from build123d import *

# Parameters (mm, degrees)
SKETCH_W  = 50.56
SKETCH_H  = 128.5
SKETCH_R  = 1.6
PAD_DEPTH = 2


with BuildPart() as part:
    # Sketch → Pad (new body)
    with BuildSketch(Plane.XZ):
        Rectangle(SKETCH_W, SKETCH_H)
        with Locations((-17.78, 61.25)):
            Circle(SKETCH_R, mode=Mode.SUBTRACT)
        with Locations((17.78, 61.25)):
            Circle(SKETCH_R, mode=Mode.SUBTRACT)
        with Locations((17.78, -61.25)):
            Circle(SKETCH_R, mode=Mode.SUBTRACT)
        with Locations((-17.78, -61.25)):
            Circle(SKETCH_R, mode=Mode.SUBTRACT)
    extrude(amount=PAD_DEPTH)


solid = part.part
Here's how the part is built. I have some questions about the finished solid (model axes, mm). Round coordinates to 2 decimals unless told otherwise and drop trailing zeros. Order: outer loops, then holes, each group sorted by start corner. A loop starts at its lowest first (then second) coordinate and runs counter-clockwise, first axis right, second up. Notation, with made-up numbers: (6.25, 6) -> (28.25, 6) arc R17 ccw to (28.25, 14) -> close; hole circle Ø5 at (-20.5, -23). An arc over 180 degrees is marked (long way). Use CSV: the item, a comma, the result in double quotes.
1. I want a section at A-A on z = -61.25. List the corners of the cut face in (x, y) for me.
Recorded:
outline,"(-25.28, -2) -> (-19.38, -2) -> (-19.38, 0) -> (-25.28, 0) -> close; (-16.18, -2) -> (16.18, -2) -> (16.18, 0) -> (-16.18, 0) -> close; (19.38, -2) -> (25.28, -2) -> (25.28, 0) -> (19.38, 0) -> close"
2. I need wall thicknesses on line 1 along Z through (x, y) = (17.78, -1.3); line 2 along Z through (x, y) = (-17, -1.6). Which ranges of each line are inside material? Lowest first, please.
Recorded:
line 1,"z = -64.25 to -62.85, -59.65 to 59.65, 62.85 to 64.25"
line 2,"z = -64.25 to -62.65, -59.85 to 59.85, 62.65 to 64.25"
3. I want a section at B-B on x = 17.78. List the corners of the cut face in (y, z) for me, and give its area (3 significant figures).
Recorded:
outline,"(-2, -64.25) -> (0, -64.25) -> (0, -62.85) -> (-2, -62.85) -> close; (-2, -59.65) -> (0, -59.65) -> (0, 59.65) -> (-2, 59.65) -> close; (-2, 62.85) -> (0, 62.85) -> (0, 64.25) -> (-2, 64.25) -> close"
area,"244 mm2"
4. Thinking about a two-plate mould opening in X: for faces 1 (the face through (17.572, -0.986, 62.836)), 2 (the face through (0, 0, 1)), which applies, pulls with the +X half, pulls with the -X half, needs draft (parallel to the pull), parting line crosses it, or undercut?
Recorded:
face 1,"undercut"
face 2,"needs draft"
